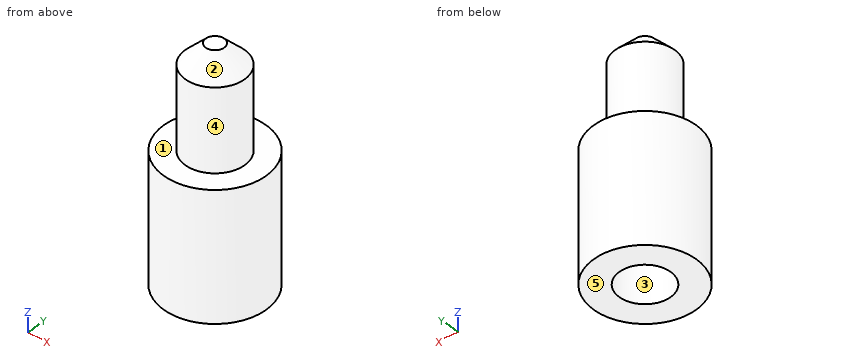
from build123d import *

# Parameters (mm, degrees)
SKETCH_1_R      = 2.5
EXTRUDE_1_DEPTH = 6.24
SKETCH_2_R      = 1.45
EXTRUDE_2_DEPTH = 5
M3X0_51_D       = 2.5
M3X0_51_DEPTH   = 5
M3X0_51_TIP     = 0.751075774
CHAMFER_1_SIZE  = 1


with BuildPart() as part:
    # Эскиз1 → Бобышка-Вытянуть1 (new body)
    with BuildSketch(Plane.XY):
        with Locations(Location((0, 0, 0), (0, 0, 180))):
            Circle(SKETCH_1_R)
    extrude(amount=EXTRUDE_1_DEPTH)

    # Эскиз2 → Бобышка-Вытянуть2 (add)
    with BuildSketch(Plane.XY.offset(6.24)):
        Circle(SKETCH_2_R)
    extrude(amount=EXTRUDE_2_DEPTH)

    # Отверстие обработанное метчиком M3x0.51
    with Locations(Plane(origin=(0, 0, 0), x_dir=(-1, 0, 0), z_dir=(0, 0, -1))):
        with Locations((0, 0)):
            Hole(M3X0_51_D / 2, depth=M3X0_51_DEPTH)
            with Locations((0, 0, -(M3X0_51_DEPTH + M3X0_51_TIP / 2))):  # 118° drill point
                Cone(0, M3X0_51_D / 2, M3X0_51_TIP, mode=Mode.SUBTRACT)

    # Фаска1
    chamfer_1_edges = [part.edges().sort_by_distance(p)[0] for p in [
        (-1.45, 0, 11.24),
    ]]
    chamfer(chamfer_1_edges, length=CHAMFER_1_SIZE)


solid = part.part
The model under review builds one solid part; all positions refer to its coordinate system, in mm. Face numbers are marked on the shaded views. A direction names the side the tool comes from. Round coordinates to 2 decimals unless told otherwise and drop trailing zeros. Write each loop counter-clockwise with the first axis right and the second up, starting at its lowest first coordinate (ties: lowest second). Pieces come first, ordered by that corner, then holes. Notation, with made-up numbers: (59, -15) -> (85, -15) arc R32 ccw to (85, 17) -> close; hole circle Ø8 at (-10.5, 36.25). An arc over 180 degrees is marked (long way). Answer as a JSON object with one key per item and string values.
1. We need section A-A on z = 2.5. State the section outline as (x, y) points, and give its area (3 significant figures).
Results found:
{"outline": "circle Ø5 at (0, 0); hole circle Ø2.5 at (0, 0)", "area": "14.7 mm^2"}
2. We need section C-C on x = -1.6. State the section outline as (y, z) points.
Results found:
{"outline": "(-1.92, 0) -> (1.92, 0) -> (1.92, 6.24) -> (-1.92, 6.24) -> close"}
3. Machinability: for the marked faces 4 and 5, which of the approach directions +Z, -Z, +X, -X, +Y, -Y give a long, thin tool a straight path to every point of the face, cutting with its end or side? Answer none if there is none.
Results found:
{"face 4": "+Z", "face 5": "-Z, +X, -X, +Y, -Y"}
4. Clearance check with flat-ended pins moving along their axes: pin 1 (1 mm diameter, centred on x = 1.5, z = 8, fed in from -Y); pin 2 (2 mm diameter, centred on y = -1.5, z = 2, fed in from +X); pin 3 (1 mm diameter, centred on y = 1, z = 9.5, fed in from -X). State where each tip first meets the part, or that it passes through.
Results found:
{"pin 1": "stops at y = -1.05", "pin 2": "stops at x = 2.45", "pin 3": "stops at x = -1.36"}
5. We need section B-B on z = 7.25. State the section outline as (x, y) points, and give its area (3 significant figures).
Results found:
{"outline": "circle Ø2.9 at (0, 0)", "area": "6.61 mm^2"}
6. The part is to be moulded in two halves that separate along X. For the marked faces 1, 2 and 3, say which applies: pulls with the +X half, pulls with the -X half, needs draft (parallel to the pull), parting line crosses it, or undercut.
Results found:
{"face 1": "needs draft", "face 2": "parting line crosses it", "face 3": "undercut"}
7. We need section D-D on y = 2.15. State the section outline as (x, z) points, and give its area (3 significant figures).
Results found:
{"outline": "(-1.28, 0) -> (1.28, 0) -> (1.28, 6.24) -> (-1.28, 6.24) -> close", "area": "15.9 mm^2"}
8. To check wall thickness, follow line 1 along Y through (x, z) = (0, 1.5); line 2 along Z through (x, y) = (-1.5, -1.1); line 3 along X through (y, z) = (0.5, 2.25). State the ranges of each line that lie inside material, in increasing order.
Results found:
{"line 1": "y = -2.5 to -1.25, 1.25 to 2.5", "line 2": "z = 0 to 6.24", "line 3": "x = -2.45 to -1.15, 1.15 to 2.45"}
